from build123d import *
from OCP.BRepFilletAPI import BRepFilletAPI_MakeFillet

# Parameters (mm, degrees)
SKETCH1_R           = 2.627
BOSS_EXTRUDE1_DEPTH = 6
BOSS_EXTRUDE2_START = -5.08
SKETCH1_3_W         = 38.1
SKETCH1_3_H         = 5.999999938
BOSS_EXTRUDE2_DEPTH = 24.13
SKETCH3_R           = 1.25
CUT_EXTRUDE1_DEPTH  = 44.944503594
FILLET1_R1          = 2.54
FILLET1_R2          = 5.08
SKETCH4_R           = 4.2145
SKETCH4_R_2         = 2.627
BOSS_EXTRUDE3_DEPTH = 2.54
BOSS_EXTRUDE4_START = 7.62
SKETCH4_2_R         = 4.2145
SKETCH4_2_R_2       = 2.627
BOSS_EXTRUDE4_DEPTH = 2.54
CHAMFER2_SIZE       = 2.54


with BuildPart() as part:
    # Sketch1 → Boss-Extrude1 (new body)
    with BuildSketch(Plane(origin=(5.08, 0, 0), x_dir=(0, 0, -1), z_dir=(1, 0, 0))):
        Polygon((-19.05, 0), (-19.05, -10.16), (0, -25.4), (19.05, -10.16), (19.05, 0), align=None)
        with Locations((0, -16.51)):
            Circle(SKETCH1_R, mode=Mode.SUBTRACT)
    boss_extrude1 = extrude(amount=BOSS_EXTRUDE1_DEPTH)

    # Sketch1<3> → Boss-Extrude2 (add)
    with BuildSketch(Plane(origin=(5.08, 0, 0), x_dir=(0, 0, -1), z_dir=(1, 0, 0)).offset(BOSS_EXTRUDE2_START)):
        with Locations((0, 2.999999969)):
            Rectangle(SKETCH1_3_W, SKETCH1_3_H)
    boss_extrude2 = extrude(amount=BOSS_EXTRUDE2_DEPTH)

    # Sketch3 → Cut-Extrude1 (cut, through all)
    with BuildSketch(Plane(origin=(0, 5.999999938, 0), x_dir=(1, 0, 0), z_dir=(0, 1, 0))):
        with Locations(Location((17.78, 12.7, 0), (0, 0, 270))):
            Circle(SKETCH3_R)
        with Locations(Location((17.78, -12.7, 0), (0, 0, 90))):
            Circle(SKETCH3_R)
    cut_extrude1 = extrude(amount=-CUT_EXTRUDE1_DEPTH, mode=Mode.SUBTRACT)

    # Mirror2: Boss-Extrude2, Cut-Extrude1 across plane
    add(boss_extrude2.mirror(Plane(origin=(0, 0, 0), x_dir=(0, 0, 1), z_dir=(1, 0, 0))))
    add(cut_extrude1.mirror(Plane(origin=(0, 0, 0), x_dir=(0, 0, 1), z_dir=(1, 0, 0))), mode=Mode.SUBTRACT)

    # Mirror3: Boss-Extrude1 across plane
    add(boss_extrude1.mirror(Plane(origin=(0, 0, 0), x_dir=(0, 0, 1), z_dir=(1, 0, 0))))

    # Fillet1: one fillet with a radius per group of edges: ONE call of the kernel's fillet builder (fillet() takes one radius for all edges)
    fillet1_edges_1 = [part.edges().sort_by_distance(p)[0] for p in [
        (8.08, -10.16, 19.05),
        (8.08, -10.16, -19.05),
        (11.08, 0, 0),
        (24.13, 2.999999969, 19.05),
        (24.13, 2.999999969, -19.05),
        (-24.13, 2.999999969, -19.05),
        (-24.13, 2.999999969, 19.05),
        (-8.08, -10.16, -19.05),
        (-8.08, -10.16, 19.05),
        (-5.08, 0, 0),
        (-11.08, 0, 0),
        (5.08, 0, 0),
    ]]
    fillet1_edges_2 = [part.edges().sort_by_distance(p)[0] for p in [
        (8.08, -25.4, 0),
        (-8.08, -25.4, 0),
    ]]
    fillet1 = BRepFilletAPI_MakeFillet(part.part.solid().wrapped)
    for e in fillet1_edges_1:
        fillet1.Add(FILLET1_R1, e.wrapped)
    for e in fillet1_edges_2:
        fillet1.Add(FILLET1_R2, e.wrapped)
    add(Compound.cast(fillet1.Shape()), mode=Mode.REPLACE)

    # Sketch4 → Boss-Extrude3 (add)
    with BuildSketch(Plane.ZY.offset(-5.08)):
        with Locations(Location((0, -16.51, 0), (0, 0, 180))):
            Circle(SKETCH4_R)
        with Locations((0, -16.51)):
            Circle(SKETCH4_R_2, mode=Mode.SUBTRACT)
    extrude(amount=BOSS_EXTRUDE3_DEPTH)

    # Sketch4<2> → Boss-Extrude4 (add)
    with BuildSketch(Plane.ZY.offset(-5.08).offset(BOSS_EXTRUDE4_START)):
        with Locations(Location((0, -16.51, 0), (0, 0, 180))):
            Circle(SKETCH4_2_R)
        with Locations((0, -16.51)):
            Circle(SKETCH4_2_R_2, mode=Mode.SUBTRACT)
    extrude(amount=BOSS_EXTRUDE4_DEPTH)

    # Chamfer2
    chamfer2_edges = [part.edges().sort_by_distance(p)[0] for p in [
        (5.08, -16.51, 4.2145),
        (-5.08, -16.51, 4.2145),
    ]]
    chamfer(chamfer2_edges, length=CHAMFER2_SIZE - 0.0001)  # a hair under: the kernel refuses the full size


solid = part.part
Design review of the part built by this model. Coordinates are the model's own, in mm. A direction names the side the tool comes from. Coordinates: 2 decimals unless noted, no trailing zeros. Order: outer loops, then holes, each group sorted by start corner. A loop starts at its lowest first (then second) coordinate and runs counter-clockwise, first axis right, second up. Notation, with made-up numbers: (-11, -7) -> (37, -7) arc R6 cw to (37, 3) -> close; hole circle Ø7 at (7.5, -22.5). An arc over 180 degrees is marked (long way). One line per item, written item: value.
1) Draft analysis for pull direction X (two halves, no side actions). For faces 4 (the face through (0, 2, -19.05)), 5 (the face through (2.663, -17.813, -4.138)), 6 (the face through (-23.366, 3.042, 18.326)), 7 (the face through (11.08, -11, 0)), state which applies: +X half, -X half, draft (parallel to the pull), parting line (faces both ways), or undercut.
Output values:
face 4: draft
face 5: undercut
face 6: -X half
face 7: +X half
2) We need section D-D, the plane z = 7.5. Give the boundary of the cut face in (x, y), then the cut area to 3 significant figures.
Output values:
outline: (-24.13, 0) -> (-13.62, 0) arc R2.54 cw to (-11.08, -2.54) -> (-11.08, -19.4) -> (-5.08, -19.4) -> (-5.08, -2.54) arc R2.54 cw to (-2.54, 0) -> (2.54, 0) arc R2.54 cw to (5.08, -2.54) -> (5.08, -19.4) -> (11.08, -19.4) -> (11.08, -2.54) arc R2.54 cw to (13.62, 0) -> (24.13, 0) -> (24.13, 6) -> (-24.13, 6) -> close
area: 528 mm2
3) We need section B-B, the plane x = 17.78. Give the boundary of the cut face in (y, z), then the cut area to 3 significant figures.
Output values:
outline: (0, -19.05) -> (6, -19.05) -> (6, -13.95) -> (0, -13.95) -> close; (0, -11.45) -> (6, -11.45) -> (6, 11.45) -> (0, 11.45) -> close; (0, 13.95) -> (6, 13.95) -> (6, 19.05) -> (0, 19.05) -> close
area: 199 mm2
4) We need section C-C, the plane y = -16.51. Count the separate pieces of the cut face and the enclosed holes in it, then the cut area to 3 significant figures.
Output values:
separate pieces: 4
enclosed holes: 0
area: 233 mm2
5) Machinability: for faces 1 (the face through (4.316, -0.724, 0.267)), 2 (the face through (-2.54, -17, -3)), 3 (the face through (19, 0, 0)), which of the approach directions +Z, -Z, +X, -X, +Y, -Y give a long, thin tool a straight path to every point of the face, cutting with its end or side? Answer none if there is none.
Output values:
face 1: +Z, -Z
face 2: +Z, -Z, -Y
face 3: +Z, -Z, +X, -Y
6) To check wall thickness, follow probe 1 along Z at (x, y) = (-17.78, 1.4); probe 2 along X at (y, z) = (4.05, -12.7); probe 3 along X at (y, z) = (-4.25, -9.5). State the ranges of each line that lie inside material, in increasing order. Write a range as [from, to].
Output values:
probe 1: z = [-19.05, -13.95], [-11.45, 11.45], [13.95, 19.05]
probe 2: x = [-24.13, -19.03], [-16.53, 16.53], [19.03, 24.13]
probe 3: x = [-11.08, -5.08], [5.08, 11.08]
7) Clearance check with flat-ended pins moving along their axes: P1, Ø6.5, axis at y = -8.5, z = -3, coming from the +X side; P2, Ø4, axis at x = 17.78, z = -12.7, coming from the +Y side; P3, Ø11.5, axis at x = 19, z = 5.5, coming from the -Y side; P4, Ø9.5, axis at y = -18.5, z = -2, coming from the -X side. State where each tip first meets the part, or that it passes through.
Output values:
P1: stops at x = 11.08
P2: stops at y = 6
P3: stops at y = -0.03
P4: stops at x = -11.08
8) We need section A-A, the plane z = 12.7. Give the boundary of the cut face in (x, y).
Output values:
outline: (-24.13, 0) -> (-19.03, 0) -> (-19.03, 6) -> (-24.13, 6) -> close; (-16.53, 0) -> (-13.62, 0) arc R2.54 cw to (-11.08, -2.54) -> (-11.08, -15.24) -> (-5.08, -15.24) -> (-5.08, -2.54) arc R2.54 cw to (-2.54, 0) -> (2.54, 0) arc R2.54 cw to (5.08, -2.54) -> (5.08, -15.24) -> (11.08, -15.24) -> (11.08, -2.54) arc R2.54 cw to (13.62, 0) -> (16.53, 0) -> (16.53, 6) -> (-16.53, 6) -> close; (19.03, 0) -> (24.13, 0) -> (24.13, 6) -> (19.03, 6) -> close
